Design review of the part shown in the three views and the two pictorial views. Dimensions are in mm from the part's minimum x, y and z. Round coordinates to 2 decimals unless told otherwise and drop trailing zeros. Loops run counter-clockwise (first coordinate to the right, second up) from the corner with the lowest first, then second, coordinate; pieces in that order, holes last. Notation, with made-up numbers: (-20, 18.25) -> (18, 18.25) arc R23 ccw to (18, 52.25) -> close; hole circle Ø1 at (-5, 48). An arc over 180 degrees is marked (long way). One line per question, with ' | ' between items. Start each with the question number.
1. For pin 1 Ø1.5 at (x, y) = (19.9, 25) entering from -Z, flat-tipped, find the tip position at first contact; note if it passes through.
2. Consider section B-B (z = 8). Write out the cut boundary in (x, y), and give its area (3 significant figures).
3. Wall thickness on line 1 along X through (y, z) = (25, 5.75); line 2 along Y through (x, z) = (19.9, 4); line 3 along Y through (x, z) = (10.4, 3.5): over which ranges is each line inside the solid? List them lowest first.
4. Consider section A-A (x = 19.9). Write out the cut boundary in (y, z), and give its area (3 significant figures).
5. Consider section D-D (x = 10.4). Write out the cut boundary in (y, z).
6. Draft analysis for pull direction X (two halves, no side actions). For the marked faces 1, 2, 3 and 4, state which applies: pulls with the +X half, pulls with the -X half, needs draft (parallel to the pull), parting line crosses it, or undercut.
7. Consider section C-C (y = 25). Write out the cut boundary in (x, z).
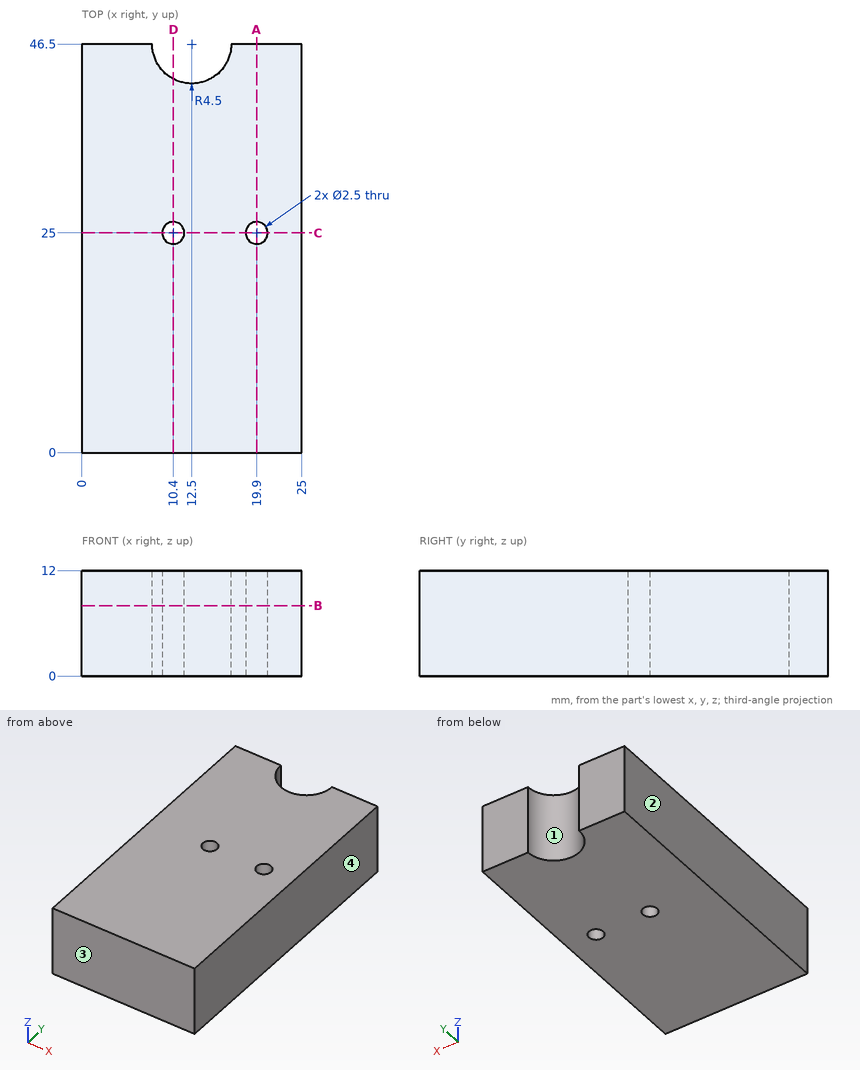
Answer block:
1) pin 1: passes through
2) outline: (0, 0) -> (25, 0) -> (25, 46.5) -> (17, 46.5) arc R4.5 cw to (8, 46.5) -> (0, 46.5) -> close; hole circle Ø2.5 at (10.4, 25); hole circle Ø2.5 at (19.9, 25) | area: 1,120 mm2
3) line 1: x = 0 to 9.15, 11.65 to 18.65, 21.15 to 25 | line 2: y = 0 to 23.75, 26.25 to 46.5 | line 3: y = 0 to 23.75, 26.25 to 42.52
4) outline: (0, 0) -> (23.75, 0) -> (23.75, 12) -> (0, 12) -> close; (26.25, 0) -> (46.5, 0) -> (46.5, 12) -> (26.25, 12) -> close | area: 528 mm2
5) outline: (0, 0) -> (23.75, 0) -> (23.75, 12) -> (0, 12) -> close; (26.25, 0) -> (42.52, 0) -> (42.52, 12) -> (26.25, 12) -> close
6) face 1: undercut | face 2: pulls with the -X half | face 3: needs draft | face 4: pulls with the +X half
7) outline: (0, 0) -> (9.15, 0) -> (9.15, 12) -> (0, 12) -> close; (11.65, 0) -> (18.65, 0) -> (18.65, 12) -> (11.65, 12) -> close; (21.15, 0) -> (25, 0) -> (25, 12) -> (21.15, 12) -> close
